Part model, mm, in its own coordinate system. A direction names the side the tool comes from. Give positions to 0.01 mm unless a question says otherwise; leave off trailing zeros. Write each loop counter-clockwise with the first axis right and the second up, starting at its lowest first coordinate (ties: lowest second). Pieces come first, ordered by that corner, then holes.
from build123d import *

# Parameters (mm, degrees)
SKETCH_1_W          = 57
SKETCH_1_H          = 16
EXTRUDE_1_DEPTH     = 5
FILLET_1_R          = 1.5
CUT_EXTRUDE_1_DEPTH = 15
HOLE_WIZARD_M41_D   = 4.5
CHAMFER_1_SIZE      = 1.5
EXTRUDE_2_DEPTH     = 6
SKETCH_9_R          = 2.25
CUT_EXTRUDE_2_DEPTH = 9.25
EXTRUDE_START       = 0.1
SKETCH_10_R         = 4
SKETCH_10_R_2       = 2.25
EXTRUDE_3_DEPTH     = 0.1


with BuildPart() as part:
    # Эскиз1 → Бобышка-Вытянуть1 (new body)
    with BuildSketch(Plane(origin=(0, 0, 0), x_dir=(1, 0, 0), z_dir=(0, 1, 0))):
        with Locations((28.5, 8)):
            Rectangle(SKETCH_1_W, SKETCH_1_H)
    extrude(amount=EXTRUDE_1_DEPTH)

    # Скругление1
    fillet_1_edges = [part.edges().sort_by_distance(p)[0] for p in [
        (28.5, 5, -16),
        (0, 5, -8),
        (28.5, 5, 0),
        (57, 5, -8),
        (0, 2.5, 0),
        (0, 2.5, -16),
        (57, 2.5, -16),
        (57, 2.5, 0),
    ]]
    fillet(fillet_1_edges, radius=FILLET_1_R)

    # Эскиз2 → Вырез-Вытянуть1 (cut)
    with BuildSketch(Plane(origin=(0, 5, 0), x_dir=(1, 0, 0), z_dir=(0, 1, 0))):
        with BuildLine():
            Line((36.175, 9.850844402), (36.175, 6.149155598))
            ThreePointArc((36.175, 6.149155598), (41.25, 8), (36.175, 9.850844402))
        make_face()
        with BuildLine():
            Line((20.825, 9.850844402), (20.825, 6.149155598))
            ThreePointArc((20.825, 6.149155598), (15.75, 8), (20.825, 9.850844402))
        make_face()
    extrude(amount=-CUT_EXTRUDE_1_DEPTH, mode=Mode.SUBTRACT)

    # Отверстие с зазором M41 (through all)
    with Locations(Plane(origin=(0, 5, 0), x_dir=(1, 0, 0), z_dir=(0, 1, 0))):
        with Locations((6.25, 8), (50.75, 8)):
            Hole(HOLE_WIZARD_M41_D / 2)

    # Фаска1
    chamfer_1_edges = [part.edges().sort_by_distance(p)[0] for p in [
        (53, 5, -8),
        (8.5, 5, -8),
    ]]
    chamfer(chamfer_1_edges, length=CHAMFER_1_SIZE)

    # Эскиз8 → Бобышка-Вытянуть2 (add)
    with BuildSketch(Plane.XZ):
        with BuildLine():
            Line((38.5, -2.5), (18.5, -2.5))
            ThreePointArc((18.5, -2.5), (13, -8), (18.5, -13.5))
            Line((18.5, -13.5), (38.5, -13.5))
            ThreePointArc((38.5, -13.5), (44, -8), (38.5, -2.5))
        make_face()
        with BuildLine():
            Line((36.175, -6.149155598), (36.175, -9.850844402))
            ThreePointArc((36.175, -9.850844402), (41.25, -8), (36.175, -6.149155598))
        make_face(mode=Mode.SUBTRACT)
        with BuildLine():
            Line((20.825, -9.850844402), (20.825, -6.149155598))
            ThreePointArc((20.825, -6.149155598), (15.75, -8), (20.825, -9.850844402))
        make_face(mode=Mode.SUBTRACT)
    extrude(amount=EXTRUDE_2_DEPTH)

    # Эскиз9 → Вырез-Вытянуть2 (cut)
    with BuildSketch(Plane.XZ.offset(6)):
        with Locations(Location((28.5, -8, 0), (0, 0, 270))):
            Circle(SKETCH_9_R)
    extrude(amount=-CUT_EXTRUDE_2_DEPTH, mode=Mode.SUBTRACT)

    # Эскиз10 → Бобышка-Вытянуть3 (add)
    with BuildSketch(Plane.XZ.offset(6).offset(EXTRUDE_START)):
        with Locations(Location((28.5, -8, 0), (0, 0, 270))):
            Circle(SKETCH_10_R)
        with Locations(Location((28.5, -8, 0), (0, 0, 270))):
            Circle(SKETCH_10_R_2, mode=Mode.SUBTRACT)
    extrude(amount=-EXTRUDE_3_DEPTH)


solid = part.part
1) 3-axis set-ups, long thin cutter, end or side, ignore diameter. For faces 1 (the flat face through (32, -6, -5)), 2 (the flat face through (36.175, 0, -8)), 3 (the cylindrical face through (13, -3, -8)), 4 (the flat face through (28, -3, -13.5)), 5 (the flat face through (27, -6.1, -10)): which of +Z, -Z, +X, -X, +Y, -Y reach the whole face in a straight line?
Check result:
face 1: -Y
face 2: +Y, -Y
face 3: -X, -Y
face 4: -Z, +X, -X, -Y
face 5: +Z, -Z, +X, -X, -Y
2) Saw through at B-B (y = -1). Write the cut outline in (x, z) (3 decimals), and give its area (3 significant figures).
Check result:
outline: (18.5, -13.5) - (38.5, -13.5) arc R5.5 ccw to (38.5, -2.5) - (18.5, -2.5) arc R5.5 ccw to start; hole (20.825, -9.851) - (20.825, -6.149) arc R2.875 ccw (long way) to start; hole circle Ø4.5 at (28.5, -8); hole (36.175, -9.851) arc R2.875 ccw (long way) to (36.175, -6.149) - close
area: 251 mm2
3) Saw through at C-C (y = 1.75). Write the cut outline in (x, z) (3 decimals), and give its area (3 significant figures).
Check result:
outline: (0, -14.5) arc R1.5 ccw to (1.5, -16) - (55.5, -16) arc R1.5 ccw to (57, -14.5) - (57, -1.5) arc R1.5 ccw to (55.5, 0) - (1.5, 0) arc R1.5 ccw to (0, -1.5) - close; hole circle Ø4.5 at (6.25, -8); hole (20.825, -9.851) - (20.825, -6.149) arc R2.875 ccw (long way) to start; hole circle Ø4.5 at (28.5, -8); hole (36.175, -9.851) arc R2.875 ccw (long way) to (36.175, -6.149) - close; hole circle Ø4.5 at (50.75, -8)
area: 814 mm2
4) Mould opens along X. For faces 6 (the cylindrical face through (56.57, 4.55, -8.09)), 7 (the cylindrical face through (26.304, -1.49, -7.512)), 8 (the cylindrical face through (0.43, 1.77, -15.55)) say: +X half, -X half, draft (parallel to the pull), parting line (faces both ways), or undercut.
Check result:
face 6: +X half
face 7: undercut
face 8: -X half
5) Saw through at A-A (x = 6.25). Write the cut outline in (y, z), and give its area (3 significant figures).
Check result:
outline: (0, -16) - (3.5, -16) arc R1.5 ccw to (5, -14.5) - (5, -11.75) - (3.5, -10.25) - (0, -10.25) - close; (0, -5.75) - (3.5, -5.75) - (5, -4.25) - (5, -1.5) arc R1.5 ccw to (3.5, 0) - (0, 0) - close
area: 54.3 mm2
6) Flat gauge pins, fed straight in: P1, Ø1.8, axis at x = 25.5, y = -4.5, coming from the -Z side; P2, Ø8, axis at x = 23.5, z = -4, coming from the -Y side; P3, Ø5, axis at x = 6.25, z = -8, coming from the +Y side; P4, Ø6, axis at x = 44, z = -10, coming from the -Y side. Where does each tip first touch, or does it go through?
Check result:
P1: stops at z = -13.5
P2: stops at y = -6.1
P3: stops at y = 3.75
P4: stops at y = -6
7) Saw through at D-D (z = -8). State how many separate pieces and enclosed holes the cut face has, and give its area (3 significant figures).
Check result:
separate pieces: 5
enclosed holes: 0
area: 268 mm2
8) Drill centre lines: L1, parallel to X at y = -2, z = -8 (3 decimals); L2, parallel to X at y = 1.6, z = -8 (3 decimals); L3, parallel to Z at x = 50.75, y = 1.7. Where is each one in solid material? Low to high.
Check result:
L1: x = 13 to 15.75, 20.825 to 26.25, 30.75 to 36.175, 41.25 to 44
L2: x = 0 to 4, 8.5 to 15.75, 20.825 to 26.25, 30.75 to 36.175, 41.25 to 48.5, 53 to 57
L3: z = -16 to -10.25, -5.75 to 0
